For this review, take the finished solid that the model builds, in its own axes (mm). Face numbers are marked on the shaded views. A direction names the side the tool comes from. Round coordinates to 2 decimals unless told otherwise and drop trailing zeros. Write each loop counter-clockwise with the first axis right and the second up, starting at its lowest first coordinate (ties: lowest second). Pieces come first, ordered by that corner, then holes.
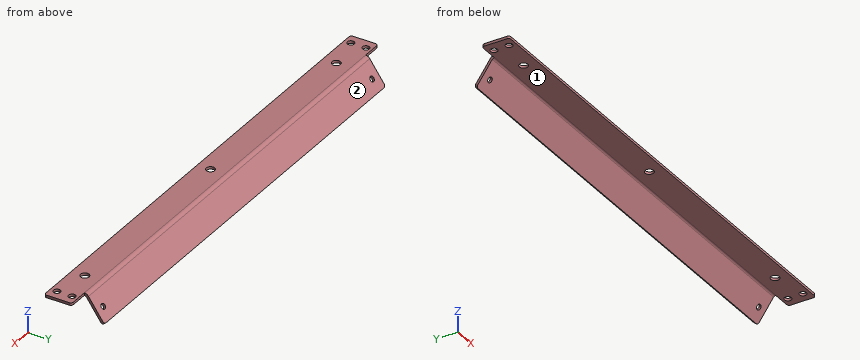
from build123d import *

# Parameters (mm, degrees)
BASE_FLANGE1_DEPTH = 638.175
SKETCH6_R          = 4.3688
SKETCH6_R_2        = 5.3578125
SKETCH6_W          = 25.4
SKETCH6_H          = 25.158862996
CUT_EXTRUDE1_DEPTH = 642.835460144
SKETCH8_R          = 3.429
CUT_EXTRUDE2_DEPTH = 3.175
FILLET1_R          = 3.175


# Sheet-metal steps are written as plain solids
with BuildPart() as part:
    # Sketch1 → Base-Flange1 (new body)
    with BuildSketch(Plane(origin=(0, 0, 0), x_dir=(0, 0, -1), z_dir=(1, 0, 0))):
        with BuildLine():
            Line((0, 0), (0, 34.794399229))
            ThreePointArc((0, 34.794399229), (0.717481209, 37.726502923), (2.707789629, 39.99601471))
            Line((2.707789629, 39.99601471), (31.209692887, 59.953262225))
            Line((31.209692887, 59.953262225), (33.030798073, 57.352454484))
            Line((33.030798073, 57.352454484), (4.528894815, 37.39520697))
            ThreePointArc((4.528894815, 37.39520697), (3.533740605, 36.260451076), (3.175, 34.794399229))
            Line((3.175, 34.794399229), (3.175, 0))
            Line((3.175, 0), (0, 0))
        make_face()
    extrude(amount=BASE_FLANGE1_DEPTH)

    # Sketch6 → Cut-Extrude1 (cut, through all)
    with BuildSketch(Plane.XY):
        with Locations((31.75, 27.305)):
            Circle(SKETCH6_R)
        with Locations((31.75, 8.255)):
            Circle(SKETCH6_R)
        with Locations((625.475, 27.305)):
            Circle(SKETCH6_R)
        with Locations((625.475, 8.255)):
            Circle(SKETCH6_R)
        with Locations((74.6125, 16.69209113)):
            Circle(SKETCH6_R_2)
        with Locations((328.6125, 16.69209113)):
            Circle(SKETCH6_R_2)
        with Locations((582.6125, 16.69209113)):
            Circle(SKETCH6_R_2)
        Polygon((19.05, 34.794399229), (44.45, 34.794399229), (44.45, 59.953262225), (0, 59.953262225), (0, 0), (19.05, 0), align=None)
        with Locations((625.475, 47.373830727)):
            Rectangle(SKETCH6_W, SKETCH6_H)
    extrude(amount=-CUT_EXTRUDE1_DEPTH, mode=Mode.SUBTRACT)

    # Sketch8 → Cut-Extrude2 (cut)
    with BuildSketch(Plane(origin=(0, 25.56548373, 17.901144426), x_dir=(1, 0, 0), z_dir=(0, 0.8191520442889929, 0.5735764363510447))):
        with Locations(Location((57.15, 44.078262225, 0), (0, 0, 270))):
            Circle(SKETCH8_R)
        with Locations(Location((600.456, 44.078262225, 0), (0, 0, 270))):
            Circle(SKETCH8_R)
    extrude(amount=-CUT_EXTRUDE2_DEPTH, mode=Mode.SUBTRACT)

    # Fillet1
    fillet1_edges = [part.edges().sort_by_distance(p)[0] for p in [
        (638.175, 34.794399229, -1.5875),
        (638.175, 0, -1.5875),
        (612.775, 58.652858355, -32.12024548),
        (19.05, 0, -1.5875),
        (44.45, 58.652858355, -32.12024548),
        (19.05, 34.794399229, -1.5875),
    ]]
    fillet(fillet1_edges, radius=FILLET1_R)


solid = part.part
(1) For pin 1 Ø12 at (y, z) = (31.5, -7) entering from +X (3 decimals); pin 2 Ø1.5 at (x, z) = (197, -12.5) entering from +Y; pin 3 Ø2 at (x, z) = (128, -5) entering from +Y; pin 4 Ø18.5 at (y, z) = (50, -8.5) entering from +X (3 decimals), all flat-tipped, find the tip position at first contact; note any pin that passes through.
Geometry check:
pin 1: stops at x = 638.175
pin 2: stops at y = 47.38
pin 3: stops at y = 42.3
pin 4: stops at x = 612.775
(2) For line 1 along X through (y, z) = (19, -2.5) (3 decimals); line 2 along Z through (x, y) = (301.5, 34) (3 decimals); line 3 along Z through (x, y) = (429, 45), list the stretches that pass through material, from the lowest coordinate up.
Geometry check:
line 1: x = 19.05 to 69.777, 79.448 to 323.777, 333.448 to 577.777, 587.448 to 638.175
line 2: z = -3.175 to 0
line 3: z = -15.39 to -9.85
(3) We need section A-A, the plane x = 301. Give the boundary of the cut face in (y, z) (3 decimals).
Geometry check:
outline: (0, -3.175) - (34.794, -3.175) arc R3.175 cw to (37.395, -4.529) - (57.352, -33.031) - (59.953, -31.21) - (39.996, -2.708) arc R6.35 ccw to (34.794, 0) - (0, 0) - close
(4) We need section B-B, the plane z = -10. Give the boundary of the cut face in (x, y) (3 decimals), and give its area (3 significant figures).
Geometry check:
outline: (44.45, 41.226) - (612.775, 41.226) - (612.775, 45.102) - (44.45, 45.102) - close
area: 2,200 mm2
(5) For the marked faces 1 and 2, list the 3-axis set-ups (+Z, -Z, +X, -X, +Y, -Y) from which the entire face can be reached by the end or side of a thin tool; tool diameter is ignored.
Geometry check:
face 1: -Z, +X, -X, -Y
face 2: +Z, +X, -X, +Y
